Geometry check sheet. Reference: drawing and pictorial views, mm from the part's lowest x, y, z. Round coordinates to 2 decimals unless told otherwise and drop trailing zeros. Write each loop counter-clockwise with the first axis right and the second up, starting at its lowest first coordinate (ties: lowest second). Pieces come first, ordered by that corner, then holes. Notation, with made-up numbers: M -30.5,47.25 L 17.5,47.25 A8 cw 17.5,51.25 Z; hole C -5.75,26 d9. An arc over 180 degrees is marked long. Put each result on its own line as item: value. Start each with the question number.
(1) Section check B-B on x = 76. Record the cut outline in (y, z).
(2) Material ranges on probe 1 along X at (y, z) = (6, 54); probe 2 along Y at (x, z) = (28.5, 78); probe 3 along X at (y, z) = (15.5, 48), recorded low to high.
(3) Section check A-A on z = 54. Record the cut outline in (x, y).
(4) Mould release check, pull along X, two halves, no side actions. Record for the marked faces 1, 2 and 3: pulls with the +X half, pulls with the -X half, needs draft (parallel to the pull), parting line crosses it, or undercut.
(5) Gauge pin test, flat ends, axial feed: pin 1 (8 mm diameter, centred on y = 20, z = 56, fed in from +X); pin 2 (5.5 mm diameter, centred on x = 76, z = 54, fed in from +Y); pin 3 (2 mm diameter, centred on x = 33.5, z = 55, fed in from +Y). Record the tip position at first contact, or that the pin passes through.
(6) Section check D-D on x = 54. Record the cut outline in (y, z), then the cut area to 3 significant figures.
(7) Section check C-C on y = 22. Record the cut outline in (x, z).
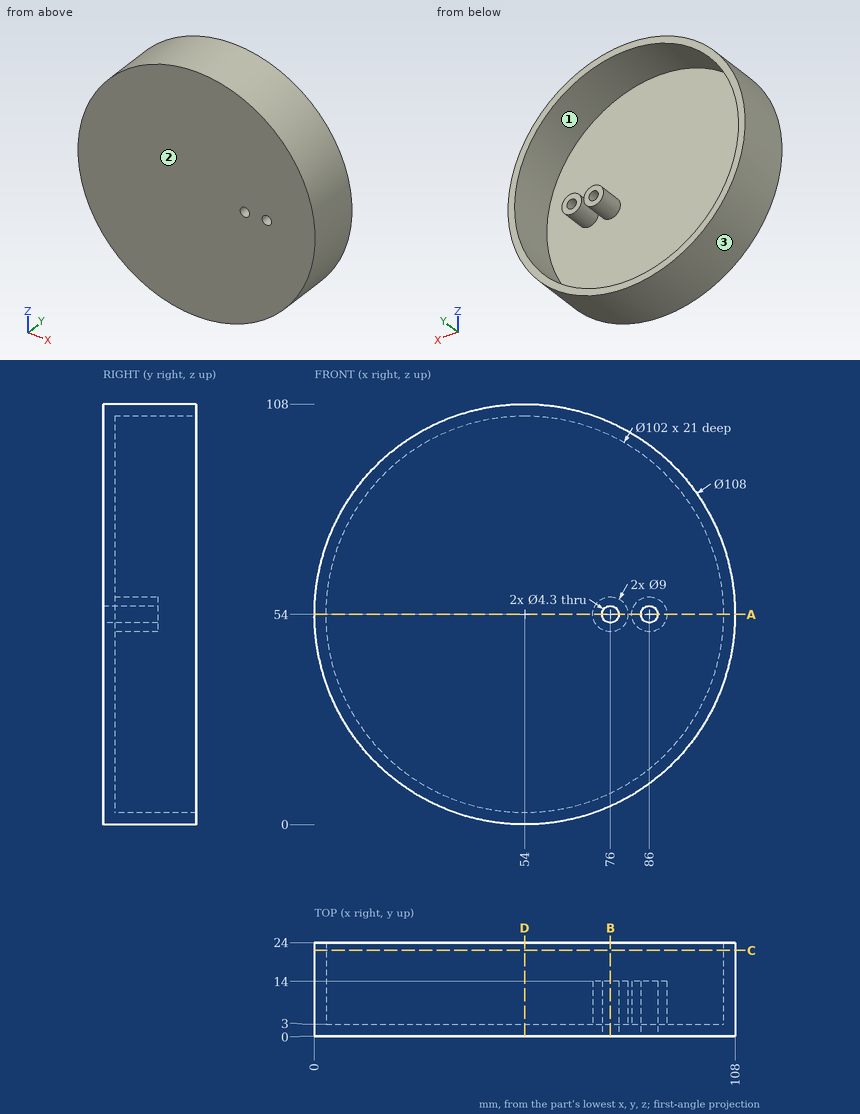
Answers follow:
1. outline: M 0,4.68 L 24,4.68 L 24,7.99 L 3,7.99 L 3,49.5 L 14,49.5 L 14,51.85 L 0,51.85 Z; M 0,56.15 L 14,56.15 L 14,58.5 L 3,58.5 L 3,100.01 L 24,100.01 L 24,103.32 L 0,103.32 Z
2. probe 1: x = 0 to 3, 71.5 to 73.85, 78.15 to 80.5, 81.5 to 83.85, 88.15 to 90.5, 105 to 108
2. probe 2: y = 0 to 3
2. probe 3: x = 0.33 to 3.35, 104.65 to 107.67
3. outline: M 0,0 L 73.85,0 L 73.85,14 L 71.5,14 L 71.5,3 L 3,3 L 3,24 L 0,24 Z; M 78.15,0 L 83.85,0 L 83.85,14 L 81.5,14 L 81.5,3 L 80.5,3 L 80.5,14 L 78.15,14 Z; M 88.15,0 L 108,0 L 108,24 L 105,24 L 105,3 L 90.5,3 L 90.5,14 L 88.15,14 Z
4. face 1: undercut
4. face 2: needs draft
4. face 3: parting line crosses it
5. pin 1: stops at x = 108
5. pin 2: stops at y = 14
5. pin 3: stops at y = 3
6. outline: M 0,0 L 24,0 L 24,3 L 3,3 L 3,105 L 24,105 L 24,108 L 0,108 Z
6. area: 450 mm^2
7. outline: C 54,54 d108; hole C 54,54 d102
